Build history of the part. All positions in model axes, mm. A direction names the side the tool comes from. Round coordinates to 2 decimals unless told otherwise and drop trailing zeros. Write each loop counter-clockwise with the first axis right and the second up, starting at its lowest first coordinate (ties: lowest second). Pieces come first, ordered by that corner, then holes. Notation, with made-up numbers: M 68,22 L 85,22 A30 cw 85,51 Z; hole C -0.5,55.5 d4. An arc over 180 degrees is marked long. Use a Markdown table: item, result.
from build123d import *

# Parameters (mm, degrees)
SKETCH1_W           = 65
SKETCH1_H           = 26
BOSS_EXTRUDE1_DEPTH = 5
SKETCH2_R           = 2.75
CUT_EXTRUDE1_DEPTH  = 5
SKETCH3_W           = 3
SKETCH3_H           = 8
BOSS_EXTRUDE2_DEPTH = 5
CHAMFER1_SIZE       = 0.8
SKETCH4_R           = 1.9
CUT_EXTRUDE2_DEPTH  = 5
CHAMFER2_SIZE       = 0.4


with BuildPart() as part:
    # Sketch1 → Boss-Extrude1 (new body)
    with BuildSketch(Plane.XY):
        with Locations((32.5, 13)):
            Rectangle(SKETCH1_W, SKETCH1_H)
    extrude(amount=BOSS_EXTRUDE1_DEPTH)

    # Sketch2 → Cut-Extrude1 (cut)
    with BuildSketch(Plane.XY.offset(5)):
        with Locations((32.5, 8)):
            Circle(SKETCH2_R)
    extrude(amount=-CUT_EXTRUDE1_DEPTH, mode=Mode.SUBTRACT)

    # Sketch3 → Boss-Extrude2 (add)
    with BuildSketch(Plane.XY.offset(5)):
        with Locations((22.75, 22)):
            Rectangle(SKETCH3_W, SKETCH3_H)
        with Locations((42.25, 22)):
            Rectangle(SKETCH3_W, SKETCH3_H)
    extrude(amount=BOSS_EXTRUDE2_DEPTH)

    # Chamfer1
    chamfer1_edges = [part.edges().sort_by_distance(p)[0] for p in [
        (21.25, 22, 10),
        (22.75, 18, 10),
        (24.25, 22, 10),
        (22.75, 26, 10),
        (40.75, 22, 10),
        (42.25, 18, 10),
        (43.75, 22, 10),
        (42.25, 26, 10),
    ]]
    chamfer(chamfer1_edges, length=CHAMFER1_SIZE)

    # Sketch4 → Cut-Extrude2 (cut)
    with BuildSketch(Plane(origin=(0, 0, 0), x_dir=(-1, 0, 0), z_dir=(0, 0, -1))):
        with Locations((-55.5, 13)):
            Circle(SKETCH4_R)
        with Locations((-9.5, 13)):
            Circle(SKETCH4_R)
    extrude(amount=-CUT_EXTRUDE2_DEPTH, mode=Mode.SUBTRACT)

    # Chamfer2
    chamfer2_edges = [part.edges().sort_by_distance(p)[0] for p in [
        (29.75, 8, 0),
        (32.5, 26, 0),
        (65, 13, 0),
        (32.5, 0, 0),
        (0, 13, 0),
        (57.4, 13, 0),
        (11.4, 13, 0),
    ]]
    chamfer(chamfer2_edges, length=CHAMFER2_SIZE)


solid = part.part
Q1. Drop flat-ended pins along their axis: P1, Ø1.5, axis at x = 42, z = 6.5, coming from the -Y side; P2, Ø12, axis at x = 14, y = 4, coming from the +Z side; P3, Ø4.5, axis at x = 55.5, y = 13, coming from the -Z side. Give the stop position or say it passes through.
Response values:
| item | result |
|---|---|
| P1 | stops at y = 18 |
| P2 | stops at z = 5 |
| P3 | stops at z = 0.05 |
Q2. Cut at B-B on y = 13. Give the cut face in (x, z).
Response values:
| item | result |
|---|---|
| outline | M 0,0.4 L 0.4,0 L 7.2,0 L 7.6,0.4 L 7.6,5 L 0,5 Z; M 11.4,0.4 L 11.8,0 L 53.2,0 L 53.6,0.4 L 53.6,5 L 11.4,5 Z; M 57.4,0.4 L 57.8,0 L 64.6,0 L 65,0.4 L 65,5 L 57.4,5 Z |
Q3. Cut at D-D on z = 1.5. Give the cut face in (x, y), and give its area (3 significant figures).
Response values:
| item | result |
|---|---|
| outline | M 0,0 L 65,0 L 65,26 L 0,26 Z; hole C 9.5,13 d3.8; hole C 32.5,8 d5.5; hole C 55.5,13 d3.8 |
| area | 1,640 mm2 |
Q4. Which spindle directions (+Z, -Z, +X, -X, +Y, -Y) get a long thin tool onto all of the face, cutting with end or side? Do faces 4 (the flat face through (43.75, 22, 7)), 5 (the flat face through (42, 18, 7)), 6 (the flat face through (32, 26, 3)), 7 (the flat face through (42, 22, 10)), 8 (the flat face through (24.25, 22, 7)). Say none if no direction does.
Response values:
| item | result |
|---|---|
| face 4 | +Z, +X, +Y, -Y |
| face 5 | +Z, +X, -X, -Y |
| face 6 | +Z, -Z, +X, -X, +Y |
| face 7 | +Z, +X, -X, +Y, -Y |
| face 8 | +Z, +Y, -Y |
Q5. Two-plate mould, pull along Y, no slides. Class faces 1 (the flat face through (21.25, 22, 7)), 2 (the flat face through (23, 18, 7)), 3 (the cylindrical face through (29.753, 8.121, 2.732)): +Y half, -Y half, draft (parallel to the pull), parting line (faces both ways), or undercut.
Response values:
| item | result |
|---|---|
| face 1 | draft |
| face 2 | -Y half |
| face 3 | undercut |
Q6. Cut at A-A on z = 5.75. Give the cut face in (x, y), and give its area (3 significant figures).
Response values:
| item | result |
|---|---|
| outline | M 21.25,18 L 24.25,18 L 24.25,26 L 21.25,26 Z; M 40.75,18 L 43.75,18 L 43.75,26 L 40.75,26 Z |
| area | 48.0 mm2 |
Q7. Drill centre lines: L1, parallel to Y at x = 32.5, z = 4; L2, parallel to Y at x = 55.5, z = 2.2; L3, parallel to Z at x = 38, y = 13.75. Where is each one in solid material? Low to high.
Response values:
| item | result |
|---|---|
| L1 | y = 0 to 5.25, 10.75 to 26 |
| L2 | y = 0 to 11.1, 14.9 to 26 |
| L3 | z = 0 to 5 |
Q8. Cut at C-C on x = 9.5. Give the cut face in (y, z), and give its area (3 significant figures).
Response values:
| item | result |
|---|---|
| outline | M 0,0.4 L 0.4,0 L 10.7,0 L 11.1,0.4 L 11.1,5 L 0,5 Z; M 14.9,0.4 L 15.3,0 L 25.6,0 L 26,0.4 L 26,5 L 14.9,5 Z |
| area | 111 mm2 |
